Here's how the part is built. I have some questions about the finished solid (model axes, mm). Round coordinates to 2 decimals unless told otherwise and drop trailing zeros. Order: outer loops, then holes, each group sorted by start corner. A loop starts at its lowest first (then second) coordinate and runs counter-clockwise, first axis right, second up.
Solid Edge part; units mm, degrees
sketch "Sketch1" plane through (0, 0, 0) normal (0, 0, 1) x (1, 0, 0)
  line L0 (22.8, 0) -> (22.8, 23.4)
  line L1 (22.8, 23.4) -> (0, 23.4)
  line L2 (0, 23.4) -> (0, 0)
  line L3 (0, 0) -> (22.8, 0)
extrude "Protrusion1" add sketch "Sketch1" along normal blind 1.6
sketch "Sketch2" plane through (11.4, 11.7, 1.6) normal (0, 0, 1) x (1, 0, 0)
  circle A0 centre (-8.22, 8.025) radius 1.875
  circle A1 centre (8.225, 8.025) radius 1.875
  circle A2 centre (-8.22, -8.02) radius 1.875
  circle A3 centre (8.225, -8.02) radius 1.875
extrude "Cutout1" cut sketch "Sketch2" against normal up to next
sketch "Sketch3" plane through (11.4, 11.7, 1.6) normal (0, 0, 1) x (1, 0, 0)
  line L0 (2.5, -2) -> (-2.5, -2)
  line L1 (-2.5, -2) -> (-2.5, 2)
  line L2 (-2.5, 2) -> (2.5, 2)
  line L3 (2.5, 2) -> (2.5, -2)
extrude "ProtrusiónExtruida_2" add sketch "Sketch3" along normal blind 1.6
fillet "Redondeo_1" radius 3 4 edges at (22.8, 0, 0.8) (22.8, 23.4, 0.8) (0, 0, 0.8) (0, 23.4, 0.8)
sketch "Sketch4" plane through (11.4, 11.7, 1.6) normal (0, 0, 1) x (1, 0, 0)
  line L0 (5.3953, 4.7) -> (9.3953, 4.7)
  line L1 (9.3953, 4.7) -> (9.3953, 3.2)
  line L2 (9.3953, 3.2) -> (5.3953, 3.2)
  line L3 (5.3953, 3.2) -> (5.3953, 4.7)
  line L4 (9.3953, 0) -> (5.3953, 0)
  line L5 (5.3953, 0) -> (5.3953, 1.5)
  line L6 (5.3953, 1.5) -> (9.3953, 1.5)
  line L7 (9.3953, 1.5) -> (9.3953, 0)
  line L8 (5.3953, -1.7) -> (9.3953, -1.7)
  line L9 (9.3953, -1.7) -> (9.3953, -3.2)
  line L10 (9.3953, -3.2) -> (5.3953, -3.2)
  line L11 (5.3953, -3.2) -> (5.3953, -1.7)
  line L12 (-9.4, 3.2) -> (-5.4, 3.2)
  line L13 (-5.4, 3.2) -> (-5.4, 4.7)
  line L14 (-5.4, 4.7) -> (-9.4, 4.7)
  line L15 (-9.4, 4.7) -> (-9.4, 3.2)
  line L16 (-9.4, 1.5) -> (-5.4, 1.5)
  line L17 (-5.4, 1.5) -> (-5.4, 0)
  line L18 (-5.4, 0) -> (-9.4, 0)
  line L19 (-9.4, 0) -> (-9.4, 1.5)
  line L20 (-9.4, -1.7) -> (-5.4, -1.7)
  line L21 (-5.4, -1.7) -> (-5.4, -3.2)
  line L22 (-5.4, -3.2) -> (-9.4, -3.2)
  line L23 (-9.4, -3.2) -> (-9.4, -1.7)
extrude "ProtrusiónExtruida_3" add sketch "Sketch4" along normal blind 0.55
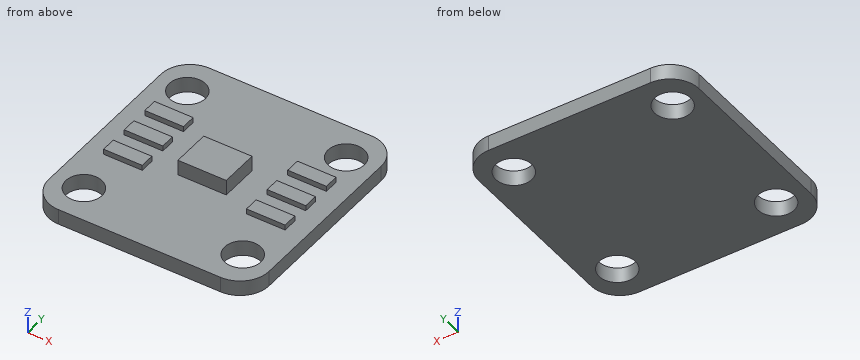
1. I'm going to push flat-ended pins straight in: P1, Ø0.6, axis at x = 3, z = 2, coming from the -Y side; P2, Ø0.8, axis at x = 18, y = 12, coming from the +Z side; P3, Ø1.3, axis at x = 11.5, z = 3, coming from the +Y side. Where does each tip first touch, or does it pass through?
Evaluation:
P1: stops at y = 8.5
P2: stops at z = 2.15
P3: stops at y = 13.7
2. If we section it at B-B, the plane x = 2.5: Write out the boundary of the cut face in (y, z).
Evaluation:
outline: (0.04, 0) - (1.93, 0) - (1.93, 1.6) - (0.04, 1.6) - close; (5.43, 0) - (17.98, 0) - (17.98, 1.6) - (16.4, 1.6) - (16.4, 2.15) - (14.9, 2.15) - (14.9, 1.6) - (13.2, 1.6) - (13.2, 2.15) - (11.7, 2.15) - (11.7, 1.6) - (10, 1.6) - (10, 2.15) - (8.5, 2.15) - (8.5, 1.6) - (5.43, 1.6) - close; (21.47, 0) - (23.36, 0) - (23.36, 1.6) - (21.47, 1.6) - close
3. If we section it at D-D, the plane y = 18.75: Write out the boundary of the cut face in (x, z).
Evaluation:
outline: (0, 0) - (1.58, 0) - (1.58, 1.6) - (0, 1.6) - close; (4.78, 0) - (18.02, 0) - (18.02, 1.6) - (4.78, 1.6) - close; (21.23, 0) - (22.8, 0) - (22.8, 1.6) - (21.23, 1.6) - close
4. I need wall thicknesses on probe 1 along X at (y, z) = (19.75, 1.3); probe 2 along Y at (x, z) = (3.18, 0.8) (3 decimals); probe 3 along Y at (x, z) = (18.25, 1.7). Which ranges of each line are inside material? Lowest first, please.
Evaluation:
probe 1: x = 0 to 1.31, 5.05 to 17.75, 21.5 to 22.8
probe 2: y = 0 to 1.805, 5.555 to 17.85, 21.6 to 23.4
probe 3: y = 8.5 to 10, 11.7 to 13.2, 14.9 to 16.4
5. If we section it at C-C, the plane x = 10: Write out the boundary of the cut face in (y, z), and give its area (3 significant figures).
Evaluation:
outline: (0, 0) - (23.4, 0) - (23.4, 1.6) - (13.7, 1.6) - (13.7, 3.2) - (9.7, 3.2) - (9.7, 1.6) - (0, 1.6) - close
area: 43.8 mm2
6. If we section it at A-A, the plane y = 3.68: Write out the boundary of the cut face in (x, z) (3 decimals).
Evaluation:
outline: (0, 0) - (1.305, 0) - (1.305, 1.6) - (0, 1.6) - close; (5.055, 0) - (17.75, 0) - (17.75, 1.6) - (5.055, 1.6) - close; (21.5, 0) - (22.8, 0) - (22.8, 1.6) - (21.5, 1.6) - close
